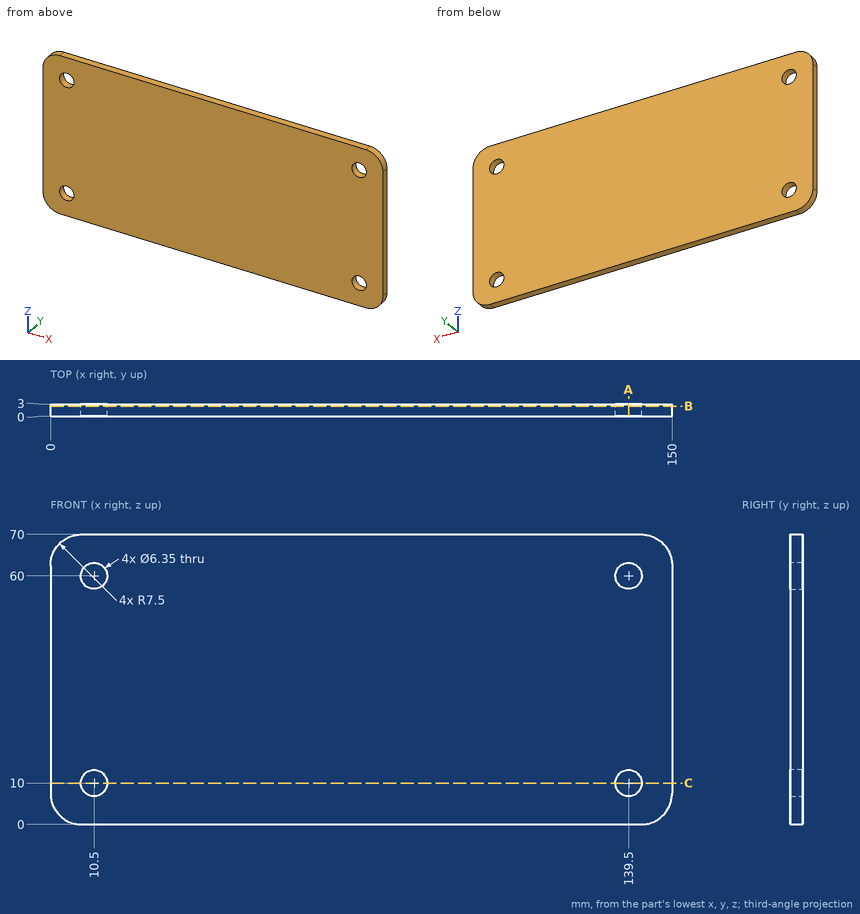
Drawing for the job (mm, zero at the part's lowest x, y, z). Give positions to 0.01 mm unless a question says otherwise; leave off trailing zeros. Order: outer loops, then holes, each group sorted by start corner. A loop starts at its lowest first (then second) coordinate and runs counter-clockwise, first axis right, second up. Notation, with made-up numbers: (72, -5.75) - (78, -5.75) arc R5 ccw to (78, 1.25) - close; hole circle Ø2 at (-16, -24). An arc over 180 degrees is marked (long way). Write item = value, one per line. Start each with the question number.
1. Cut at C-C, the plane z = 10. List the corners of the cut face in (x, y) (3 decimals).
2. Cut at A-A, the plane x = 139.5. List the corners of the cut face in (y, z) (3 decimals), and give its area (3 significant figures).
3. Cut at B-B, the plane y = 2.5. List the corners of the cut face in (x, z) (3 decimals), and give its area (3 significant figures).
4. Probe line 1 along X through (y, z) = (1.5, 10) (3 decimals); line 2 along Z through (x, y) = (141.5, 0.2); line 3 along Z through (x, y) = (13, 1.4). List the from-to ranges inside material, lowest first.
5. Drop a flat-ended pin along its axis: P1, Ø4, axis at x = 10.5, z = 60, coming from the +Y side. Give the stop position or say it passes through.
Taken from the geometry:
q1.outline = (0, 0) - (7.325, 0) - (7.325, 3) - (0, 3) - close; (13.675, 0) - (136.325, 0) - (136.325, 3) - (13.675, 3) - close; (142.675, 0) - (150, 0) - (150, 3) - (142.675, 3) - close
q2.outline = (0, 0) - (3, 0) - (3, 6.825) - (0, 6.825) - close; (0, 13.175) - (3, 13.175) - (3, 56.825) - (0, 56.825) - close; (0, 63.175) - (3, 63.175) - (3, 70) - (0, 70) - close
q2.area = 172 mm²
q3.outline = (0, 7.5) arc R7.5 ccw to (7.5, 0) - (142.5, 0) arc R7.5 ccw to (150, 7.5) - (150, 62.5) arc R7.5 ccw to (142.5, 70) - (7.5, 70) arc R7.5 ccw to (0, 62.5) - close; hole circle Ø6.35 at (10.5, 10); hole circle Ø6.35 at (10.5, 60); hole circle Ø6.35 at (139.5, 10); hole circle Ø6.35 at (139.5, 60)
q3.area = 10,300 mm²
q4.line_1 = 0 to 7.325, 13.675 to 136.325, 142.675 to 150
q4.line_2 = 0 to 7.53, 12.47 to 57.53, 62.47 to 70
q4.line_3 = 0 to 8.04, 11.96 to 58.04, 61.96 to 70
q5.P1 = through
